from build123d import *

# Parameters (mm, degrees)
ENLEV_MAT_EXTRU_1_DEPTH = 1
ESQUISSE3_W             = 2
ESQUISSE3_H             = 10
CHANFREIN1_SIZE         = 0.4
ENL_V_MAT_EXTRU_1_DEPTH = 1


with BuildPart() as part:
    # Esquisse1 → Base-R_volution (revolve)
    with BuildSketch(Plane(origin=(0, 0, 0), x_dir=(1, 0, 0), z_dir=(0, 1, 0)), mode=Mode.PRIVATE) as base_r_volution_sk:
        with BuildLine():
            Line((0, 0), (3.35, 0))
            Line((3.35, 0), (3.349988656, 1.349988656))
            ThreePointArc((3.349988656, 1.349988656), (3.314559619, 1.541470155), (3.210770724, 1.706237405))
            ThreePointArc((3.210770724, 1.706237405), (1.651042147, 2.288775714), (0, 2.503633679))
            Line((0, 2.503633679), (0, 0))
        make_face()
    revolve(base_r_volution_sk.sketch.rotate(Axis((0, 0, 0), (0, 0, -1)), 180), axis=Axis((0, 0, 0), (0, 0, -1)))

    # Esquisse2 → Enlev. mat.-Extru.1 (cut)
    with BuildSketch(Plane.XY.offset(-3.1)):
        Polygon((0.6, -0.6), (0.6, -2.35), (-0.6, -2.35), (-0.6, -0.6), (-2.35, -0.6), (-2.35, 0.6), (-0.6, 0.6), (-0.6, 2.35), (0.6, 2.35), (0.6, 0.6), (2.35, 0.6), (2.35, -0.6), align=None)
    extrude(amount=ENLEV_MAT_EXTRU_1_DEPTH, mode=Mode.SUBTRACT)

    # Esquisse3 → Boss.-R_vol.1 (revolve)
    with BuildSketch(Plane(origin=(0, 0, 0), x_dir=(1, 0, 0), z_dir=(0, 1, 0)), mode=Mode.PRIVATE) as boss_r_vol_1_sk:
        with Locations((1, -5)):
            Rectangle(ESQUISSE3_W, ESQUISSE3_H)
    revolve(boss_r_vol_1_sk.sketch.rotate(Axis((0, 0, 0), (0, 0, 1)), 15.212714494), axis=Axis((0, 0, 0), (0, 0, 1)))

    # Chanfrein1
    chanfrein1_edges = [part.edges().sort_by_distance(p)[0] for p in [
        (-1.929916577, -0.524806638, 10),
    ]]
    chamfer(chanfrein1_edges, length=CHANFREIN1_SIZE)

    # Esquisse6 → Enl_v. mat.-Extru.1 (cut)
    with BuildSketch(Plane(origin=(0, 0, -2.1), x_dir=(-1, 0, 0), z_dir=(0, 0, -1))):
        with BuildLine():
            Line((2.206431589, 0.6), (0.6, 0.6))
            Line((0.6, 0.6), (0.6, 2.206431589))
            ThreePointArc((0.6, 2.206431589), (0, 2.286556441), (-0.6, 2.206431589))
            Line((-0.6, 2.206431589), (-0.6, 0.6))
            Line((-0.6, 0.6), (-2.206431589, 0.6))
            ThreePointArc((-2.206431589, 0.6), (-2.286556441, 0), (-2.206431589, -0.6))
            Line((-2.206431589, -0.6), (-0.6, -0.6))
            Line((-0.6, -0.6), (-0.6, -2.206431589))
            ThreePointArc((-0.6, -2.206431589), (0, -2.286556441), (0.6, -2.206431589))
            Line((0.6, -2.206431589), (0.6, -0.6))
            Line((0.6, -0.6), (2.206431589, -0.6))
            ThreePointArc((2.206431589, -0.6), (2.286556441, 0), (2.206431589, 0.6))
        make_face()
    extrude(amount=-ENL_V_MAT_EXTRU_1_DEPTH, mode=Mode.SUBTRACT)


solid = part.part
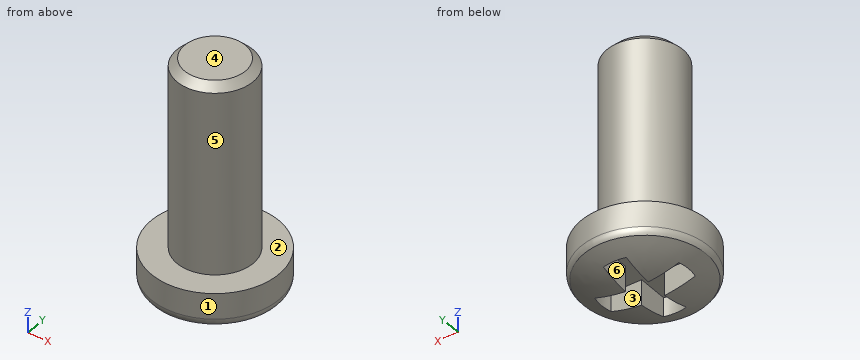
Part model, mm, in its own coordinate system. Face numbers are marked on the shaded views. A direction names the side the tool comes from. Coordinates: 2 decimals unless noted, no trailing zeros. Loops run counter-clockwise (first coordinate to the right, second up) from the corner with the lowest first, then second, coordinate; pieces in that order, holes last. Notation, with made-up numbers: (-39.5, 20) -> (-4.5, 20) arc R16 cw to (-4.5, 37) -> close; hole circle Ø8 at (8, 49.25). An arc over 180 degrees is marked (long way). Use a Markdown table: item, result. Add a question column.
Item 1: Pull direction Y, two halves, no side cores. Call the marked faces 1, 2 and 3: +Y half, -Y half, draft (parallel to the pull), parting line (faces both ways), or undercut.
Item 2: Band-saw the part on A-A on z = -0.75. Write the cut outline in (x, y).
Item 3: Flat gauge pins, fed straight in: P1, Ø1.1, axis at x = 2, z = -2, coming from the -Y side; P2, Ø1.5, axis at y = -1, z = -2, coming from the -X side; P3, Ø0.7, axis at x = 1.5, z = -1.5, coming from the +Y side. Where does each tip first touch, or does it go through?
Item 4: Band-saw the part on B-B on z = 0.5. Write the cut outline in (x, y).
Item 5: Probe probe 1 along Z at (x, y) = (-1, 0.25); probe 2 along Y at (x, z) = (1.25, -1.5); probe 3 along Z at (x, y) = (1.75, -2.5). List the from-to ranges inside material, lowest first.
Item 6: Which spindle directions (+Z, -Z, +X, -X, +Y, -Y) get a long thin tool onto all of the face, cutting with end or side? Do the marked faces 4, 5 and 6. Say none if no direction does.
Geometry says:
| question | item | result |
|---|---|---|
| 1 | face 1 | parting line |
| 1 | face 2 | draft |
| 1 | face 3 | undercut |
| 2 | outline | circle Ø6.7 at (0, 0) |
| 3 | P1 | y = -2.86 |
| 3 | P2 | x = -3.3 |
| 3 | P3 | y = 3.14 |
| 4 | outline | circle Ø4 at (0, 0) |
| 5 | probe 1 | -1.1 to 10 |
| 5 | probe 2 | -3.09 to -0.6, 0.6 to 3.09 |
| 5 | probe 3 | -1.78 to 0 |
| 6 | face 4 | +Z, +X, -X, +Y, -Y |
| 6 | face 5 | +Z |
| 6 | face 6 | -Z |
